Input: part model. Units: mm. Frame: model coordinates. A direction names the side the tool comes from. Round coordinates to 2 decimals unless told otherwise and drop trailing zeros. Order: outer loops, then holes, each group sorted by start corner. A loop starts at its lowest first (then second) coordinate and runs counter-clockwise, first axis right, second up.
Item 1: Reachability of faces 1 (the cylindrical face through (11.08, 25.85, 34.59)), 2 (the cylindrical face through (18.324, -1.172, -28.577)), 3 (the flat face through (24, -1, 1)) from +Z, -Z, +X, -X, +Y, -Y: full face, straight path, thin tool, end or side. Return the list, or none.
Item 2: Line query: L1, parallel to Y at x = 23, z = -37; L2, parallel to Y at x = 12, z = 41; L3, parallel to Z at x = 20, y = 30. Output: solid intervals per line, ascending.
Item 3: Mould query, pull axis X, two halves, no side actions, for faces 4 (the cylindrical face through (6.66, 25.95, -33.78)), 5 (the flat face through (13, 25.9, -41.4)), 6 (the cylindrical face through (8.63, -32.59, 34.59)), 7 (the cylindrical face through (14.285, 3.584, 34.587)). Classes: released by +X, released by -X, zero draft, split by the parting line, or undercut.
Item 4: Cut plane A-A on x = 4.75. Output: boundary loops of the cut face in (y, z), then the cut area to 3 significant figures.
Item 5: First-contact query: pin 1 (14.5 mm diameter, centred on y = 30, z = -37.5, fed in from -X); pin 2 (14.5 mm diameter, centred on y = -30, z = -37.5, fed in from +X); pin 3 (14.5 mm diameter, centred on y = -29.5, z = -35.5, fed in from +X). Flat tips, straight axial feed; report the tip coordinate or a pass-through.
Item 6: Cut plane B-B on z = -37.5. Give the number of separate pieces and of enclosed holes in the cut face, then the cut area to 3 significant figures.
```python
from build123d import *

# Parameters (mm, degrees)
F0_W     = 90
F0_H     = 100
F0_R     = 5.5
F1_DEPTH = 24
F2_R     = 9
F3_DEPTH = 11
F4_R     = 4.25
F5_DEPTH = 35
F6_SIZE  = 4.25
F7_SIZE  = 0.5


with BuildPart() as f1:
    # F0 (on Right) → F1 (new body)
    with BuildSketch(Plane.YZ):
        Rectangle(F0_W, F0_H)
        with Locations((-30, -37.5)):
            Circle(F0_R, mode=Mode.SUBTRACT)
        with Locations((0, -37.5)):
            Circle(F0_R, mode=Mode.SUBTRACT)
        with Locations((30, -37.5)):
            Circle(F0_R, mode=Mode.SUBTRACT)
    extrude(amount=F1_DEPTH)

    # F2 (on face) → F3 (cut)
    with BuildSketch(Plane.YZ.offset(24)):
        with Locations((-30, -37.5)):
            Circle(F2_R)
        with Locations((0, -37.5)):
            Circle(F2_R)
        with Locations((30, -37.5)):
            Circle(F2_R)
    extrude(amount=-F3_DEPTH, mode=Mode.SUBTRACT)

    # F4 (on face) → F5 (cut)
    with BuildSketch(Plane.XY.offset(50)):
        with Locations((12, -30)):
            Circle(F4_R)
        with Locations((12, 0)):
            Circle(F4_R)
        with Locations((12, 30)):
            Circle(F4_R)
    extrude(amount=-F5_DEPTH, mode=Mode.SUBTRACT)

    # F6
    f6_edges = [f1.edges().sort_by_distance(p)[0] for p in [
        (7.75, 30, 15),
        (7.75, 0, 15),
        (7.75, -30, 15),
    ]]
    chamfer(f6_edges, length=F6_SIZE)

    # F7
    f7_edges = [f1.edges().sort_by_distance(p)[0] for p in [
        (0, -35.5, -37.5),
        (0, -5.5, -37.5),
        (0, 24.5, -37.5),
        (7.75, 30, 50),
        (7.75, 0, 50),
        (7.75, -30, 50),
        (24, -39, -37.5),
        (24, -9, -37.5),
        (24, 21, -37.5),
    ]]
    chamfer(f7_edges, length=F7_SIZE)


solid = f1.part
```
From the geometry:
1. face 1: +Z
1. face 2: +X
1. face 3: +Z, -Z, +X, +Y, -Y
2. L1: y = -45 to -38.99, -21.01 to -8.99, 8.99 to 21.01, 38.99 to 45
2. L2: y = -45 to -34.25, -25.75 to -4.25, 4.25 to 25.75, 34.25 to 45
2. L3: z = -50 to -46.5, -28.5 to 50
3. face 4: zero draft
3. face 5: released by +X
3. face 6: undercut
3. face 7: undercut
4. outline: (-45, -50) - (45, -50) - (45, 50) - (-45, 50) - close; hole circle Ø11 at (-30, -37.5); hole circle Ø11 at (0, -37.5); hole circle Ø11 at (30, -37.5)
4. area: 8,710 mm2
5. pin 1: stops at x = 0
5. pin 2: stops at x = 13
5. pin 3: stops at x = 23.81
6. separate pieces: 4
6. enclosed holes: 0
6. area: 1,140 mm2
